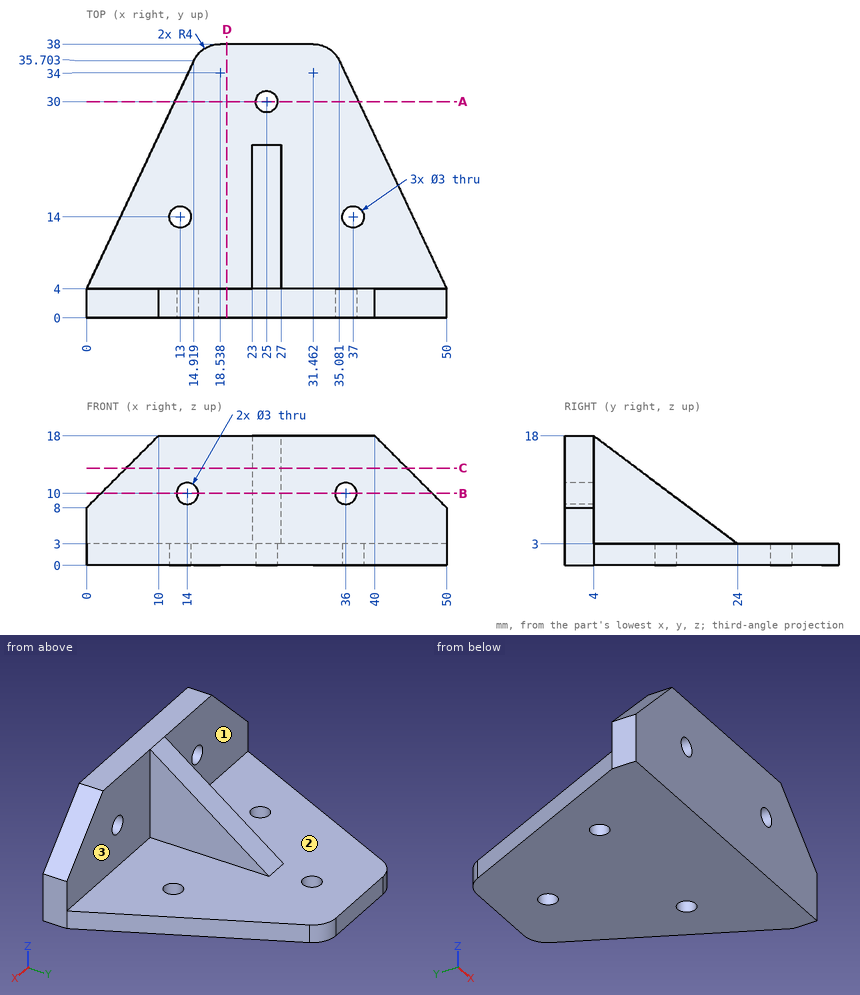
Study the drawing (mm; zero at the part's minimum x, y, z) and answer. A direction names the side the tool comes from. Give positions to 0.01 mm unless a question says otherwise; leave off trailing zeros. Order: outer loops, then holes, each group sorted by start corner. A loop starts at its lowest first (then second) coordinate and runs counter-clockwise, first axis right, second up. Notation, with made-up numbers: (34, 79.5) - (68, 79.5) arc R5 cw to (68, 85.5) - close; hole circle Ø10 at (-24.75, 79). An arc over 180 degrees is marked (long way). Answer as CSV lines item,"result". Start each with the question number.
Q1. The part is cut by section A-A (y = 30). Write down the section's boundary in (x, z) (1 decimal).
Q2. For the marked faces 1, 2 and 3, determine the directions among +Z, -Z, +X, -X, +Y, -Y from which every point of the face is accessible in a straight line to the end or side of a thin tool.
Q3. The part is cut by section D-D (x = 19.5). Write down the section's boundary in (y, z).
Q4. Find the intervals of material crossed by L1, parallel to Z at x = 36, y = 1.9; L2, parallel to X at y = 2.45, z = 10; L3, parallel to X at y = 14, z = 1.75 (1 decimal), in increasing order. Write a range as [from, to].
Q5. The part is cut by section C-C (z = 13.5). Write down the section's boundary in (x, y).
Q6. Given pin 1 Ø3 at (y, z) = (12, 12.5) entering from -X; pin 2 Ø2.5 at (x, y) = (37, 14) entering from +Z, each flat-ended and moving along its own axis, determine where each tip first touches the part or whether it passes through.
Q7. The part is cut by section B-B (z = 10). Write down the section's boundary in (x, y), then the cut area to 3 significant figures.
Check result:
1,outline,"(12.2, 0) - (23.5, 0) - (23.5, 3) - (12.2, 3) - close; (26.5, 0) - (37.8, 0) - (37.8, 3) - (26.5, 3) - close"
2,face 1,"+Z, -X, +Y"
2,face 2,"+Z, +Y"
2,face 3,"+Z, +X, +Y"
3,outline,"(0, 0) - (38, 0) - (38, 3) - (4, 3) - (4, 18) - (0, 18) - close"
4,L1,"z = [0, 8.5], [11.5, 18]"
4,L2,"x = [2, 12.5], [15.5, 34.5], [37.5, 48]"
4,L3,"x = [4.7, 11.5], [14.5, 35.5], [38.5, 45.3]"
5,outline,"(5.5, 0) - (44.5, 0) - (44.5, 4) - (27, 4) - (27, 10) - (23, 10) - (23, 4) - (5.5, 4) - close"
6,pin 1,"stops at x = 23"
6,pin 2,"passes through"
7,outline,"(2, 0) - (12.5, 0) - (12.5, 4) - (2, 4) - close; (15.5, 0) - (34.5, 0) - (34.5, 4) - (27, 4) - (27, 14.67) - (23, 14.67) - (23, 4) - (15.5, 4) - close; (37.5, 0) - (48, 0) - (48, 4) - (37.5, 4) - close"
7,area,"203 mm²"
